The listing builds one solid part. Answer for the finished solid, in the listing's coordinates (mm). Face numbers are marked on the shaded views. A direction names the side the tool comes from. Coordinates: 2 decimals unless noted, no trailing zeros. Order: outer loops, then holes, each group sorted by start corner. A loop starts at its lowest first (then second) coordinate and runs counter-clockwise, first axis right, second up. Notation, with made-up numbers: (82.5, 17) - (94.5, 17) arc R24 ccw to (94.5, 54) - close; hole circle Ø10 at (81.25, 56.25). An arc over 180 degrees is marked (long way). Use a Markdown table: item, result. Add a question column.
Item 1: The part is cut by section B-B, the plane x = -31.5. Give the vertices of the cut face in (y, z), then the cut area to 3 significant figures.
Item 2: The part is cut by section A-A, the plane z = -14. Give the vertices of the cut face in (x, y).
Item 3: The mould has two halves that part along Z. Classify the marked faces 5, 6, 7 and 8: released by +Z, released by -Z, zero draft, split by the parting line, or undercut.
Item 4: Find the intervals of material crossed by line 1 along X through (y, z) = (10.5, -15); line 2 along X through (y, z) = (15.25, 19.5); line 3 along X through (y, z) = (4.5, 59), in increasing order.
Item 5: Flat-ended cylindrical pins translate along their axes: P1, Ø11, axis at y = 12, z = 20, coming from the +X side; P2, Ø3, axis at x = -25.5, y = 5, coming from the -Z side; P3, Ø4, axis at x = -21.5, z = 36.5, coming from the +Y side. Find the tip coordinate at first contact, or state that the pin passes through.
Item 6: The part is cut by section C-C, the plane z = 18.5. Give the vertices of the cut face in (x, y), then the cut area to 3 significant figures.
Item 7: For the marked faces 1, 2, 3 and 4, determine the directions among +Z, -Z, +X, -X, +Y, -Y from which every point of the face is accessible in a straight line to the end or side of a thin tool.
Item 8: The part is cut by section D-D, the plane y = 10.75. State how many separate pieces and enclosed holes the cut face has, then the cut area to 3 significant figures.
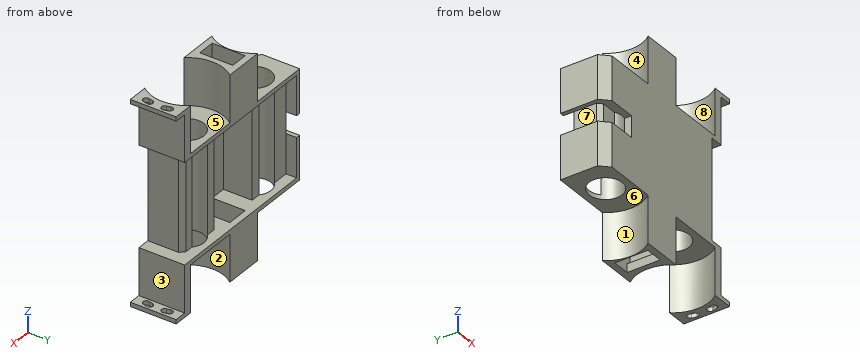
from build123d import *

# Parameters (mm, degrees)
SKETCH1_W           = 95
SKETCH1_H           = 95
BOSS_EXTRUDE1_DEPTH = 25
SKETCH2_R           = 7.75
CUT_EXTRUDE2_DEPTH  = 100
SKETCH3_R           = 17
CUT_EXTRUDE3_DEPTH  = 22
CUT_EXTRUDE4_START  = -22
SKETCH4_R           = 17
CUT_EXTRUDE4_DEPTH  = 22
SKETCH5_W           = 6.246993927
SKETCH5_H           = 25
CUT_EXTRUDE5_DEPTH  = 22
SKETCH6_W           = 7.178723585
SKETCH6_H           = 25
CUT_EXTRUDE6_DEPTH  = 22
SKETCH8_W           = 99.503929421
SKETCH8_H           = 3.5
CUT_EXTRUDE7_DEPTH  = 100
SKETCH9_W           = 8.3
SKETCH9_H           = 15.5
CUT_EXTRUDE11_DEPTH = 100
SKETCH13_W          = 87
SKETCH13_H          = 15.5
CUT_EXTRUDE12_DEPTH = 2
SKETCH14_W          = 25.5
SKETCH14_H          = 47
CUT_EXTRUDE14_DEPTH = 18.5
SKETCH16_W          = 24.75
SKETCH16_H          = 47
CUT_EXTRUDE15_DEPTH = 5
SKETCH17_W          = 20.919567191
SKETCH17_H          = 47
CUT_EXTRUDE16_DEPTH = 5
CUT_EXTRUDE17_DEPTH = 100
FILLET6_R           = 1.5
FILLET7_R           = 1.5
FILLET8_R           = 1.5
FILLET9_R           = 1.5
SKETCH19_W          = 12.12120401
SKETCH19_H          = 21.5
CUT_EXTRUDE20_DEPTH = 100
SKETCH20_W          = 5.709228799
SKETCH20_H          = 91
CUT_EXTRUDE23_DEPTH = 100
SKETCH21_W          = 6
SKETCH21_H          = 47
CUT_EXTRUDE26_DEPTH = 40
CHAMFER1_SIZE       = 2
SKETCH22_W          = 15
SKETCH22_H          = 10
CUT_EXTRUDE27_DEPTH = 4
SKETCH23_W          = 2
SKETCH23_H          = 10
CUT_EXTRUDE28_DEPTH = 54
CHAMFER2_SIZE       = 2
CHAMFER3_SIZE       = 4
CHAMFER4_SIZE       = 4


with BuildPart() as part:
    # Sketch1 → Boss-Extrude1 (new body)
    with BuildSketch(Plane(origin=(0, 0, 0), x_dir=(1, 0, 0), z_dir=(0, 1, 0))):
        with Locations((3.271948822, -17.506298191)):
            Rectangle(SKETCH1_W, SKETCH1_H)
    extrude(amount=BOSS_EXTRUDE1_DEPTH)

    # Sketch2 → Cut-Extrude2 (cut)
    with BuildSketch(Plane.XY.offset(65.006298191)):
        with Locations((-29.228051178, 10.75)):
            Circle(SKETCH2_R)
        with Locations((15.771948822, 10.75)):
            Circle(SKETCH2_R)
    extrude(amount=-CUT_EXTRUDE2_DEPTH, mode=Mode.SUBTRACT)

    # Sketch3 → Cut-Extrude3 (cut)
    with BuildSketch(Plane.XY.offset(65.006298191)):
        with Locations((-29.228051178, 10.75)):
            Circle(SKETCH3_R)
        with Locations((15.771948822, 10.75)):
            Circle(SKETCH3_R)
    extrude(amount=-CUT_EXTRUDE3_DEPTH, mode=Mode.SUBTRACT)

    # Sketch4 → Cut-Extrude4 (cut)
    with BuildSketch(Plane(origin=(0, 0, -29.993701809), x_dir=(-1, 0, 0), z_dir=(0, 0, -1)).offset(CUT_EXTRUDE4_START)):
        with Locations((-15.771948822, 10.75)):
            Circle(SKETCH4_R)
        with Locations((29.228051178, 10.75)):
            Circle(SKETCH4_R)
    extrude(amount=CUT_EXTRUDE4_DEPTH, mode=Mode.SUBTRACT)

    # Sketch5 → Cut-Extrude5 (cut)
    with BuildSketch(Plane.XY.offset(65.006298191)):
        with Locations((-41.104554214, 12.5)):
            Rectangle(SKETCH5_W, SKETCH5_H)
    extrude(amount=-CUT_EXTRUDE5_DEPTH, mode=Mode.SUBTRACT)

    # Sketch6 → Cut-Extrude6 (cut)
    with BuildSketch(Plane(origin=(0, 0, -29.993701809), x_dir=(-1, 0, 0), z_dir=(0, 0, -1))):
        with Locations((40.638689386, 12.5)):
            Rectangle(SKETCH6_W, SKETCH6_H)
    extrude(amount=-CUT_EXTRUDE6_DEPTH, mode=Mode.SUBTRACT)

    # Sketch8 → Cut-Extrude7 (cut)
    with BuildSketch(Plane(origin=(0, 0, -29.993701809), x_dir=(-1, 0, 0), z_dir=(0, 0, -1))):
        with Locations((-1.019984112, 23.25)):
            Rectangle(SKETCH8_W, SKETCH8_H)
    extrude(amount=-CUT_EXTRUDE7_DEPTH, mode=Mode.SUBTRACT)

    # Sketch9 → Cut-Extrude11 (cut)
    with BuildSketch(Plane.XY.offset(65.006298191)):
        with Locations((-7.828051178, 10.75)):
            Rectangle(SKETCH9_W, SKETCH9_H)
    extrude(amount=-CUT_EXTRUDE11_DEPTH, mode=Mode.SUBTRACT)

    # Sketch13 → Cut-Extrude12 (cut)
    with BuildSketch(Plane.ZY.offset(3.678051178)):
        with Locations((17.506298191, 10.75)):
            Rectangle(SKETCH13_W, SKETCH13_H)
    extrude(amount=-CUT_EXTRUDE12_DEPTH, mode=Mode.SUBTRACT)

    # Sketch14 → Cut-Extrude14 (cut)
    with BuildSketch(Plane(origin=(0, 21.5, 0), x_dir=(1, 0, 0), z_dir=(0, 1, 0))):
        with Locations((-6.728051178, -17.506298191)):
            Rectangle(SKETCH14_W, SKETCH14_H)
    extrude(amount=-CUT_EXTRUDE14_DEPTH, mode=Mode.SUBTRACT)

    # Sketch16 → Cut-Extrude15 (cut)
    with BuildSketch(Plane(origin=(0, 21.5, 0), x_dir=(1, 0, 0), z_dir=(0, 1, 0))):
        with Locations((-29.853051178, -17.506298191)):
            Rectangle(SKETCH16_W, SKETCH16_H)
    extrude(amount=-CUT_EXTRUDE15_DEPTH, mode=Mode.SUBTRACT)

    # Sketch17 → Cut-Extrude16 (cut)
    with BuildSketch(Plane(origin=(0, 21.5, 0), x_dir=(1, 0, 0), z_dir=(0, 1, 0))):
        with Locations((16.481732418, -17.506298191)):
            Rectangle(SKETCH17_W, SKETCH17_H)
    extrude(amount=-CUT_EXTRUDE16_DEPTH, mode=Mode.SUBTRACT)

    # Sketch18 → Cut-Extrude17 (cut)
    with BuildSketch(Plane.XY.offset(65.006298191)):
        with BuildLine():
            Line((34.66639245, 12.75), (37.680851122, 12.75))
            ThreePointArc((37.680851122, 12.75), (37.300376381, 15.28065192), (36.628602437, 17.75))
            Line((36.628602437, 17.75), (33.435470555, 17.75))
            ThreePointArc((33.435470555, 17.75), (34.221100776, 15.291893017), (34.66639245, 12.75))
        make_face()
        with BuildLine():
            Line((34.66639245, 8.75), (37.680851122, 8.75))
            ThreePointArc((37.680851122, 8.75), (37.300376381, 6.21934808), (36.628602437, 3.75))
            Line((36.628602437, 3.75), (33.435470555, 3.75))
            ThreePointArc((33.435470555, 3.75), (34.221100776, 6.208106983), (34.66639245, 8.75))
        make_face()
    extrude(amount=-CUT_EXTRUDE17_DEPTH, mode=Mode.SUBTRACT)

    # Fillet6
    fillet6_edges = [part.edges().sort_by_distance(p)[0] for p in [
        (33.435470555, 17.75, 17.506298191),
        (36.628602437, 17.75, 17.506298191),
    ]]
    fillet(fillet6_edges, radius=FILLET6_R - 0.0001)  # a hair under: the kernel refuses the full size

    # Fillet7
    fillet7_edges = [part.edges().sort_by_distance(p)[0] for p in [
        (37.680851122, 12.75, 17.506298191),
        (34.66639245, 12.75, 17.506298191),
    ]]
    fillet(fillet7_edges, radius=FILLET7_R - 0.0001)  # a hair under: the kernel refuses the full size

    # Fillet8
    fillet8_edges = [part.edges().sort_by_distance(p)[0] for p in [
        (33.435470555, 3.75, 17.506298191),
        (36.628602437, 3.75, 17.506298191),
    ]]
    fillet(fillet8_edges, radius=FILLET8_R - 0.0001)  # a hair under: the kernel refuses the full size

    # Fillet9
    fillet9_edges = [part.edges().sort_by_distance(p)[0] for p in [
        (37.680851122, 8.75, 17.506298191),
        (34.66639245, 8.75, 17.506298191),
    ]]
    fillet(fillet9_edges, radius=FILLET9_R - 0.0001)  # a hair under: the kernel refuses the full size

    # Sketch19 → Cut-Extrude20 (cut)
    with BuildSketch(Plane.XY.offset(65.006298191)):
        with Locations((44.711346817, 10.75)):
            Rectangle(SKETCH19_W, SKETCH19_H)
    extrude(amount=-CUT_EXTRUDE20_DEPTH, mode=Mode.SUBTRACT)

    # Sketch20 → Cut-Extrude23 (cut)
    with BuildSketch(Plane(origin=(0, 21.5, 0), x_dir=(1, 0, 0), z_dir=(0, 1, 0))):
        with Locations((35.796130413, -17.506298191)):
            Rectangle(SKETCH20_W, SKETCH20_H)
    extrude(amount=-CUT_EXTRUDE23_DEPTH, mode=Mode.SUBTRACT)

    # Sketch21 → Cut-Extrude26 (cut)
    with BuildSketch(Plane(origin=(0, 21.5, 0), x_dir=(1, 0, 0), z_dir=(0, 1, 0))):
        with Locations((29.941516013, -17.506298191)):
            Rectangle(SKETCH21_W, SKETCH21_H)
    extrude(amount=-CUT_EXTRUDE26_DEPTH, mode=Mode.SUBTRACT)

    # Chamfer1
    chamfer1_edges = [part.edges().sort_by_distance(p)[0] for p in [
        (26.941516013, 16.5, 17.506298191),
    ]]
    chamfer(chamfer1_edges, length=CHAMFER1_SIZE)

    # Sketch22 → Cut-Extrude27 (cut)
    with BuildSketch(Plane(origin=(0, 0, 0), x_dir=(-1, 0, 0), z_dir=(0, -1, 0))):
        with Locations((34.728051178, -17.506298191)):
            Rectangle(SKETCH22_W, SKETCH22_H)
    extrude(amount=-CUT_EXTRUDE27_DEPTH, mode=Mode.SUBTRACT)

    # Sketch23 → Cut-Extrude28 (cut)
    with BuildSketch(Plane(origin=(0, 0, 0), x_dir=(-1, 0, 0), z_dir=(0, -1, 0))):
        with Locations((43.228051178, -17.506298191)):
            Rectangle(SKETCH23_W, SKETCH23_H)
    extrude(amount=-CUT_EXTRUDE28_DEPTH, mode=Mode.SUBTRACT)

    # Chamfer2
    chamfer2_edges = [part.edges().sort_by_distance(p)[0] for p in [
        (-42.228051178, 4, 17.506298191),
    ]]
    chamfer(chamfer2_edges, length=CHAMFER2_SIZE)

    # Chamfer3
    chamfer3_edges = [part.edges().sort_by_distance(p)[0] for p in [
        (-44.228051178, 0, 2.256298191),
    ]]
    chamfer(chamfer3_edges, length=CHAMFER3_SIZE)

    # Chamfer4
    chamfer4_edges = [part.edges().sort_by_distance(p)[0] for p in [
        (-44.228051178, 0, 32.756298191),
    ]]
    chamfer(chamfer4_edges, length=CHAMFER4_SIZE)


solid = part.part
Solution:
| question | item | result |
|---|---|---|
| 1 | outline | (0, -7.99) - (3.34, -7.99) - (3.34, 12.51) - (0, 12.51) - close; (0, 22.51) - (3.34, 22.51) - (3.34, 43.01) - (0, 43.01) - close; (18.16, -7.99) - (21.5, -7.99) - (21.5, -5.99) - (18.16, -5.99) - close; (18.16, 41.01) - (21.5, 41.01) - (21.5, 43.01) - (18.16, 43.01) - close |
| 1 | area | 150 mm2 |
| 2 | outline | (-16.06, 0) - (2.6, 0) arc R17 cw to (2.6, 21.5) - (-16.06, 21.5) arc R17 cw to start; (28.94, 0) - (32.94, 0) - (32.94, 21.5) - (28.94, 21.5) arc R17 cw to start; hole (-11.98, 3) - (-1.68, 3) - (-1.68, 18.5) - (-11.98, 18.5) - close |
| 3 | face 5 | released by +Z |
| 3 | face 6 | released by -Z |
| 3 | face 7 | undercut |
| 3 | face 8 | zero draft |
| 4 | line 1 | x = -12.23 to -11.98, -1.68 to -1.23, 32.77 to 32.94 |
| 4 | line 2 | x = -42.23 to -35.54, -22.92 to -19.48, 6.02 to 9.46, 22.08 to 26.19 |
| 4 | line 3 | x = -13.42 to -11.98, -1.68 to -0.04, 31.58 to 32.94 |
| 5 | P1 | stops at x = 26.94 |
| 5 | P2 | stops at z = -7.99 |
| 5 | P3 | stops at y = 16.5 |
| 6 | outline | (-42.23, 6) - (-40.23, 4) - (-33.04, 4) arc R7.75 cw to (-34.42, 16.5) - (-42.23, 16.5) - close; (-27.23, 0) - (26.94, 0) - (26.94, 14.5) - (24.94, 16.5) - (20.97, 16.5) arc R7.75 cw (long way) to (10.58, 16.5) - (6.02, 16.5) - (6.02, 3) - (-19.48, 3) - (-19.48, 16.5) - (-24.03, 16.5) arc R7.75 cw to (-27.23, 3.26) - close |
| 6 | area | 389 mm2 |
| 7 | face 1 | -Z, -X |
| 7 | face 2 | -Z |
| 7 | face 3 | +X, +Y, -Y |
| 7 | face 4 | +Z, -X |
| 8 | separate pieces | 4 |
| 8 | enclosed holes | 0 |
| 8 | area | 890 mm2 |
